```python
from build123d import *

# Parameters (mm, degrees)
SKETCH_1_W          = 120
SKETCH_1_H          = 60
EXTRUDE_1_DEPTH     = 5
CUT_EXTRUDE_1_REACH = 115.997
SKETCH_2_R          = 1.65
CUT_EXTRUDE_2_REACH = 115.997
SKETCH_4_R          = 1.6
CUT_EXTRUDE_3_REACH = 115.997
SKETCH_5_R          = 1.65
FILLET_1_R          = 1


with BuildPart() as part:
    # 草图1 → 凸台-拉伸1 (new body)
    with BuildSketch(Plane.XY):
        with Locations((-40, -24.5)):
            Rectangle(SKETCH_1_W, SKETCH_1_H)
    extrude(amount=EXTRUDE_1_DEPTH)

    # 草图2 → 切除-拉伸1 (cut, up to next)
    with BuildSketch(Plane.XY.offset(5), mode=Mode.PRIVATE) as cut_extrude_1_sk1:
        with Locations((-50, -13)):
            Circle(SKETCH_2_R)
    cut_extrude_1_tool1 = extrude(cut_extrude_1_sk1.sketch, amount=-CUT_EXTRUDE_1_REACH, mode=Mode.PRIVATE) & part.part
    # 草图2 → 切除-拉伸1 (cut, up to next)
    with BuildSketch(Plane.XY.offset(5), mode=Mode.PRIVATE) as cut_extrude_1_sk2:
        with Locations((-75, -24.5)):
            Circle(SKETCH_2_R)
    cut_extrude_1_tool2 = extrude(cut_extrude_1_sk2.sketch, amount=-CUT_EXTRUDE_1_REACH, mode=Mode.PRIVATE) & part.part
    # 草图2 → 切除-拉伸1 (cut, up to next)
    with BuildSketch(Plane.XY.offset(5), mode=Mode.PRIVATE) as cut_extrude_1_sk3:
        with Locations((-50, -36)):
            Circle(SKETCH_2_R)
    cut_extrude_1_tool3 = extrude(cut_extrude_1_sk3.sketch, amount=-CUT_EXTRUDE_1_REACH, mode=Mode.PRIVATE) & part.part
    add(cut_extrude_1_tool1.solids().sort_by_distance((-50, -13, 5))[0], mode=Mode.SUBTRACT)
    add(cut_extrude_1_tool2.solids().sort_by_distance((-75, -24.5, 5))[0], mode=Mode.SUBTRACT)
    add(cut_extrude_1_tool3.solids().sort_by_distance((-50, -36, 5))[0], mode=Mode.SUBTRACT)

    # 草图4 → 切除-拉伸2 (cut, up to next)
    with BuildSketch(Plane(origin=(0, 0, 0), x_dir=(-1, 0, 0), z_dir=(0, 0, -1)), mode=Mode.PRIVATE) as cut_extrude_2_sk1:
        with Locations((90, 0)):
            Circle(SKETCH_4_R)
    cut_extrude_2_tool1 = extrude(cut_extrude_2_sk1.sketch, amount=-CUT_EXTRUDE_2_REACH, mode=Mode.PRIVATE) & part.part
    # 草图4 → 切除-拉伸2 (cut, up to next)
    with BuildSketch(Plane(origin=(0, 0, 0), x_dir=(-1, 0, 0), z_dir=(0, 0, -1)), mode=Mode.PRIVATE) as cut_extrude_2_sk2:
        with Locations((70, 0)):
            Circle(SKETCH_4_R)
    cut_extrude_2_tool2 = extrude(cut_extrude_2_sk2.sketch, amount=-CUT_EXTRUDE_2_REACH, mode=Mode.PRIVATE) & part.part
    # 草图4 → 切除-拉伸2 (cut, up to next)
    with BuildSketch(Plane(origin=(0, 0, 0), x_dir=(-1, 0, 0), z_dir=(0, 0, -1)), mode=Mode.PRIVATE) as cut_extrude_2_sk3:
        with Locations((70, -49)):
            Circle(SKETCH_4_R)
    cut_extrude_2_tool3 = extrude(cut_extrude_2_sk3.sketch, amount=-CUT_EXTRUDE_2_REACH, mode=Mode.PRIVATE) & part.part
    # 草图4 → 切除-拉伸2 (cut, up to next)
    with BuildSketch(Plane(origin=(0, 0, 0), x_dir=(-1, 0, 0), z_dir=(0, 0, -1)), mode=Mode.PRIVATE) as cut_extrude_2_sk4:
        with Locations((90, -49)):
            Circle(SKETCH_4_R)
    cut_extrude_2_tool4 = extrude(cut_extrude_2_sk4.sketch, amount=-CUT_EXTRUDE_2_REACH, mode=Mode.PRIVATE) & part.part
    # 草图4 → 切除-拉伸2 (cut, up to next)
    with BuildSketch(Plane(origin=(0, 0, 0), x_dir=(-1, 0, 0), z_dir=(0, 0, -1)), mode=Mode.PRIVATE) as cut_extrude_2_sk5:
        with Locations((10, -49)):
            Circle(SKETCH_4_R)
    cut_extrude_2_tool5 = extrude(cut_extrude_2_sk5.sketch, amount=-CUT_EXTRUDE_2_REACH, mode=Mode.PRIVATE) & part.part
    # 草图4 → 切除-拉伸2 (cut, up to next)
    with BuildSketch(Plane(origin=(0, 0, 0), x_dir=(-1, 0, 0), z_dir=(0, 0, -1)), mode=Mode.PRIVATE) as cut_extrude_2_sk6:
        with Locations((-10, -49)):
            Circle(SKETCH_4_R)
    cut_extrude_2_tool6 = extrude(cut_extrude_2_sk6.sketch, amount=-CUT_EXTRUDE_2_REACH, mode=Mode.PRIVATE) & part.part
    # 草图4 → 切除-拉伸2 (cut, up to next)
    with BuildSketch(Plane(origin=(0, 0, 0), x_dir=(-1, 0, 0), z_dir=(0, 0, -1)), mode=Mode.PRIVATE) as cut_extrude_2_sk7:
        with Locations((-10, 0)):
            Circle(SKETCH_4_R)
    cut_extrude_2_tool7 = extrude(cut_extrude_2_sk7.sketch, amount=-CUT_EXTRUDE_2_REACH, mode=Mode.PRIVATE) & part.part
    # 草图4 → 切除-拉伸2 (cut, up to next)
    with BuildSketch(Plane(origin=(0, 0, 0), x_dir=(-1, 0, 0), z_dir=(0, 0, -1)), mode=Mode.PRIVATE) as cut_extrude_2_sk8:
        with Locations((10, 0)):
            Circle(SKETCH_4_R)
    cut_extrude_2_tool8 = extrude(cut_extrude_2_sk8.sketch, amount=-CUT_EXTRUDE_2_REACH, mode=Mode.PRIVATE) & part.part
    add(cut_extrude_2_tool1.solids().sort_by_distance((-90, 0, 0))[0], mode=Mode.SUBTRACT)
    add(cut_extrude_2_tool2.solids().sort_by_distance((-70, 0, 0))[0], mode=Mode.SUBTRACT)
    add(cut_extrude_2_tool3.solids().sort_by_distance((-70, -49, 0))[0], mode=Mode.SUBTRACT)
    add(cut_extrude_2_tool4.solids().sort_by_distance((-90, -49, 0))[0], mode=Mode.SUBTRACT)
    add(cut_extrude_2_tool5.solids().sort_by_distance((-10, -49, 0))[0], mode=Mode.SUBTRACT)
    add(cut_extrude_2_tool6.solids().sort_by_distance((10, -49, 0))[0], mode=Mode.SUBTRACT)
    add(cut_extrude_2_tool7.solids().sort_by_distance((10, 0, 0))[0], mode=Mode.SUBTRACT)
    add(cut_extrude_2_tool8.solids().sort_by_distance((-10, 0, 0))[0], mode=Mode.SUBTRACT)

    # 草图5 → 切除-拉伸3 (cut, up to next)
    with BuildSketch(Plane.XY.offset(5), mode=Mode.PRIVATE) as cut_extrude_3_sk1:
        with Locations((-20, -43.5)):
            Circle(SKETCH_5_R)
    cut_extrude_3_tool1 = extrude(cut_extrude_3_sk1.sketch, amount=-CUT_EXTRUDE_3_REACH, mode=Mode.PRIVATE) & part.part
    # 草图5 → 切除-拉伸3 (cut, up to next)
    with BuildSketch(Plane.XY.offset(5), mode=Mode.PRIVATE) as cut_extrude_3_sk2:
        with Locations((-20, -24.5)):
            Circle(SKETCH_5_R)
    cut_extrude_3_tool2 = extrude(cut_extrude_3_sk2.sketch, amount=-CUT_EXTRUDE_3_REACH, mode=Mode.PRIVATE) & part.part
    # 草图5 → 切除-拉伸3 (cut, up to next)
    with BuildSketch(Plane.XY.offset(5), mode=Mode.PRIVATE) as cut_extrude_3_sk3:
        with Locations((-20, -5.5)):
            Circle(SKETCH_5_R)
    cut_extrude_3_tool3 = extrude(cut_extrude_3_sk3.sketch, amount=-CUT_EXTRUDE_3_REACH, mode=Mode.PRIVATE) & part.part
    add(cut_extrude_3_tool1.solids().sort_by_distance((-20, -43.5, 5))[0], mode=Mode.SUBTRACT)
    add(cut_extrude_3_tool2.solids().sort_by_distance((-20, -24.5, 5))[0], mode=Mode.SUBTRACT)
    add(cut_extrude_3_tool3.solids().sort_by_distance((-20, -5.5, 5))[0], mode=Mode.SUBTRACT)

    # 圆角1
    fillet_1_edges = [part.edges().sort_by_distance(p)[0] for p in [
        (-100, -24.5, 5),
        (-40, -54.5, 5),
        (20, -24.5, 5),
        (-40, -54.5, 0),
        (-100, -24.5, 0),
        (-40, 5.5, 0),
        (20, -24.5, 0),
        (20, -54.5, 2.5),
        (-100, -54.5, 2.5),
        (-100, 5.5, 2.5),
        (20, 5.5, 2.5),
        (-40, 5.5, 5),
    ]]
    fillet(fillet_1_edges, radius=FILLET_1_R)


solid = part.part
```
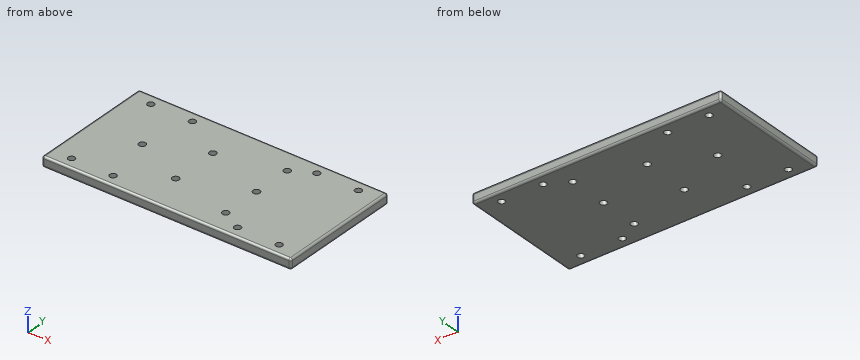
Check sheet for the modelled part. Datum: model origin and axes. Units: mm. Round coordinates to 2 decimals unless told otherwise and drop trailing zeros. Order: outer loops, then holes, each group sorted by start corner. A loop starts at its lowest first (then second) coordinate and runs counter-clockwise, first axis right, second up.
1) Scan lines: line 1 (Y direction, x = -50, z = 2.65); line 2 (Y direction, x = -51, z = 1.1); line 3 (X direction, y = -35.5, z = 0.85). Record each from-to range of solid material in increasing order.
2) Section check C-C (z = 2.1). Give the number of separate pieces and of enclosed holes in the cut face, and give its area (3 significant figures).
3) Section check A-A (x = -75). Record the boundary of the cut face in (y, z).
4) Section check B-B (y = -13). Record the boundary of the cut face in (x, z).
5) Section check D-D (x = -50). Record the boundary of the cut face in (y, z), and give its area (3 significant figures).
Result:
1. line 1: y = -54.5 to -37.65, -34.35 to -14.65, -11.35 to 5.5
1. line 2: y = -54.5 to -37.31, -34.69 to -14.31, -11.69 to 5.5
1. line 3: x = -99.99 to -51.57, -48.43 to 19.99
2. separate pieces: 1
2. enclosed holes: 14
2. area: 7,080 mm2
3. outline: (-54.5, 1) arc R1 ccw to (-53.5, 0) - (-26.15, 0) - (-26.15, 5) - (-53.5, 5) arc R1 ccw to (-54.5, 4) - close; (-22.85, 0) - (4.5, 0) arc R1 ccw to (5.5, 1) - (5.5, 4) arc R1 ccw to (4.5, 5) - (-22.85, 5) - close
4. outline: (-100, 1) arc R1 ccw to (-99, 0) - (-51.65, 0) - (-51.65, 5) - (-99, 5) arc R1 ccw to (-100, 4) - close; (-48.35, 0) - (19, 0) arc R1 ccw to (20, 1) - (20, 4) arc R1 ccw to (19, 5) - (-48.35, 5) - close
5. outline: (-54.5, 1) arc R1 ccw to (-53.5, 0) - (-37.65, 0) - (-37.65, 5) - (-53.5, 5) arc R1 ccw to (-54.5, 4) - close; (-34.35, 0) - (-14.65, 0) - (-14.65, 5) - (-34.35, 5) - close; (-11.35, 0) - (4.5, 0) arc R1 ccw to (5.5, 1) - (5.5, 4) arc R1 ccw to (4.5, 5) - (-11.35, 5) - close
5. area: 266 mm2
